Drawing for the job (mm, zero at the part's lowest x, y, z). Give positions to 0.01 mm unless a question says otherwise; leave off trailing zeros. Order: outer loops, then holes, each group sorted by start corner. A loop starts at its lowest first (then second) coordinate and runs counter-clockwise, first axis right, second up. Notation, with made-up numbers: M 74,12.5 L 84,12.5 A7 ccw 84,24.5 Z; hole C 84,37.5 d3. An arc over 180 degrees is marked long. Answer as a JSON object with one key per item and string values.
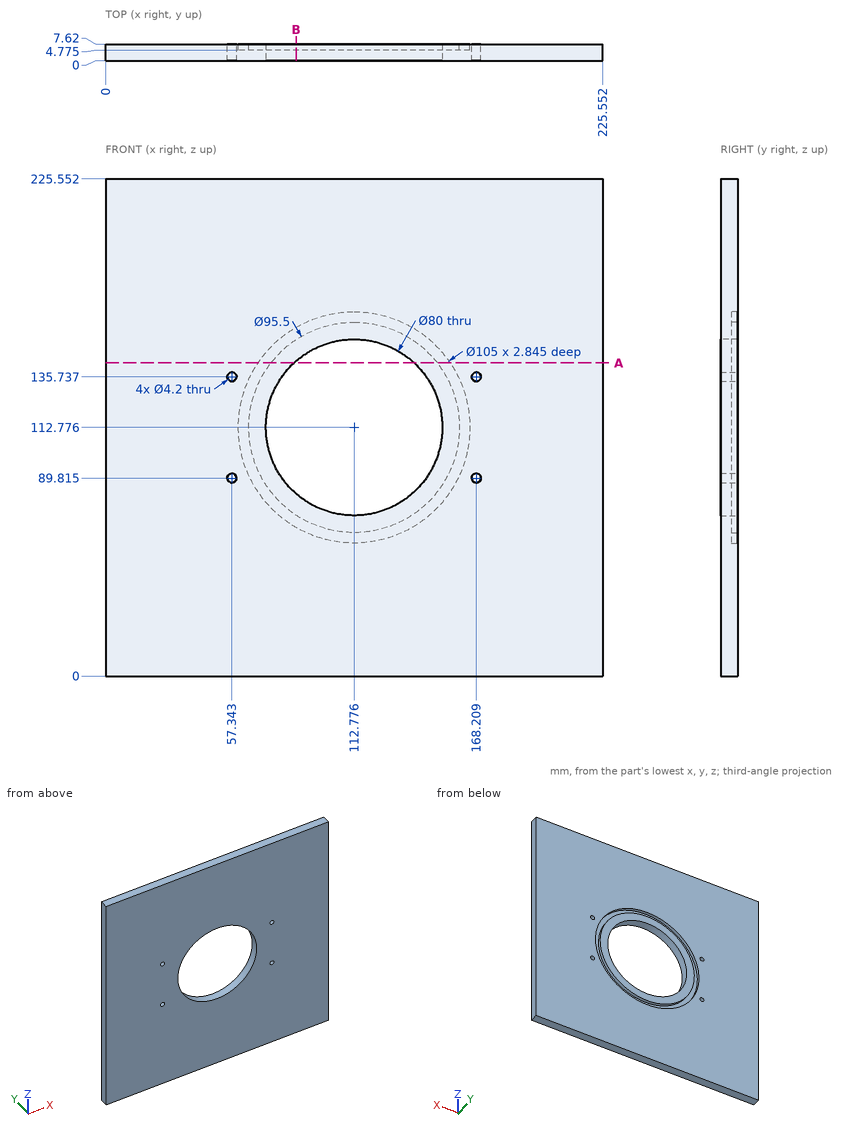
1. Probe line 1 along Z through (x, y) = (91, 5) (1 decimal); line 2 along X through (y, z) = (5.25, 102) (1 decimal); line 3 along X through (y, z) = (5, 135) (1 decimal). List the from-to ranges inside material, lowest first.
Worked answers:
{"line 1": "z = 0 to 65, 70.3 to 79.2, 146.3 to 155.3, 160.5 to 225.6", "line 2": "x = 0 to 61.4, 66.3 to 74.3, 151.3 to 159.3, 164.2 to 225.6", "line 3": "x = 0 to 55.4, 59.3 to 65.2, 70.5 to 79.5, 146 to 155, 160.3 to 166.2, 170.2 to 225.6"}
2. Cut at A-A on z = 142. Give the cut face in (x, y) (1 decimal), plus the area to 3 significant figures.
Worked answers:
{"outline": "M 0,0 L 85.5,0 L 85.5,7.6 L 75,7.6 L 75,4.8 L 69.2,4.8 L 69.2,7.6 L 0,7.6 Z; M 140.1,0 L 225.6,0 L 225.6,7.6 L 156.4,7.6 L 156.4,4.8 L 150.5,4.8 L 150.5,7.6 L 140.1,7.6 Z", "area": "1,270 mm^2"}
3. Cut at B-B on x = 86.5. Give the cut face in (y, z) (1 decimal).
Worked answers:
{"outline": "M 0,0 L 7.6,0 L 7.6,67.3 L 4.8,67.3 L 4.8,72.9 L 7.6,72.9 L 7.6,82.6 L 0,82.6 Z; M 0,142.9 L 7.6,142.9 L 7.6,152.6 L 4.8,152.6 L 4.8,158.2 L 7.6,158.2 L 7.6,225.6 L 0,225.6 Z"}
